For this review, take the finished solid that the model builds, in its own axes (mm). A direction names the side the tool comes from. Give positions to 0.01 mm unless a question says otherwise; leave off trailing zeros. Order: outer loops, then holes, each group sorted by start corner. A loop starts at its lowest first (then second) coordinate and runs counter-clockwise, first axis right, second up. Notation, with made-up numbers: (23.25, -15.75) -> (32.25, -15.75) arc R21 cw to (32.25, -1.75) -> close; hole circle Ø8 at (79, 39.25). An arc over 180 degrees is marked (long way). One line per item, written item: value. Start each with the question number.
from build123d import *

# Parameters (mm, degrees)
F0_W     = 1.5
F0_H     = 3.75
F0_W_2   = 12
F0_H_2   = 1.5
F0_H_3   = 21
F1_DEPTH = 25


with BuildPart() as f1:
    # F0 (on Front) → F1 (new body)
    with BuildSketch(Plane.XZ):
        with Locations((6.75, 46.125)):
            Rectangle(F0_W, F0_H)
        with Locations((-6.75, 46.125)):
            Rectangle(F0_W, F0_H)
        with Locations((0, 69.75)):
            Rectangle(F0_W_2, F0_H_2)
        with Locations((0, 58.5)):
            Rectangle(F0_W_2, F0_H_3)
        with Locations((0, 46.125)):
            Rectangle(F0_W_2, F0_H)
        with BuildLine():
            ThreePointArc((-6, 29.3938769134), (0, 30), (6, 29.3938769134))
            Line((6, 29.3938769134), (6, 44.25))
            Line((6, 44.25), (-6, 44.25))
            Line((-6, 44.25), (-6, 29.3938769134))
        make_face()
    extrude(amount=F1_DEPTH)


solid = f1.part
Q1. Take a section at B-B (z = 55). State the section outline as (x, y) points, and give its area (3 significant figures).
Q2. For line 1 along Z through (x, y) = (-6.5, -6.5); line 2 along Z through (x, y) = (-0.25, -14.5); line 3 along X through (y, z) = (-21.5, 64), list the stretches that pass through material, from the lowest coordinate up.
Q3. Take a section at A-A (y = -7). State the section outline as (x, z) points.
Q4. For faces 1 (the flat face through (7, -12, 44.25)), 2 (the flat face through (-6, -12, 59)), 3 (the flat face through (6, -12, 59)), list the 3-axis set-ups (+Z, -Z, +X, -X, +Y, -Y) from which the entire face can be reached by the end or side of a thin tool; tool diameter is ignored.
Q5. For pin 1 Ø12 at (y, z) = (-17.5, 37) entering from +X; pin 2 Ø0.8 at (x, y) = (-7, -10) entering from +Z; pin 3 Ø0.8 at (x, y) = (-6.5, -7) entering from -Z, all flat-tipped, find the tip position at first contact; note any pin that passes through.
Answers below:
1. outline: (-6, -25) -> (6, -25) -> (6, 0) -> (-6, 0) -> close
1. area: 300 mm²
2. line 1: z = 44.25 to 48
2. line 2: z = 30 to 70.5
2. line 3: x = -6 to 6
3. outline: (-7.5, 44.25) -> (-6, 44.25) -> (-6, 29.39) arc R30 cw to (6, 29.39) -> (6, 44.25) -> (7.5, 44.25) -> (7.5, 48) -> (6, 48) -> (6, 70.5) -> (-6, 70.5) -> (-6, 48) -> (-7.5, 48) -> close
4. face 1: -Z, +X, +Y, -Y
4. face 2: +Z, -X, +Y, -Y
4. face 3: +Z, +X, +Y, -Y
5. pin 1: stops at x = 6
5. pin 2: stops at z = 48
5. pin 3: stops at z = 44.25
